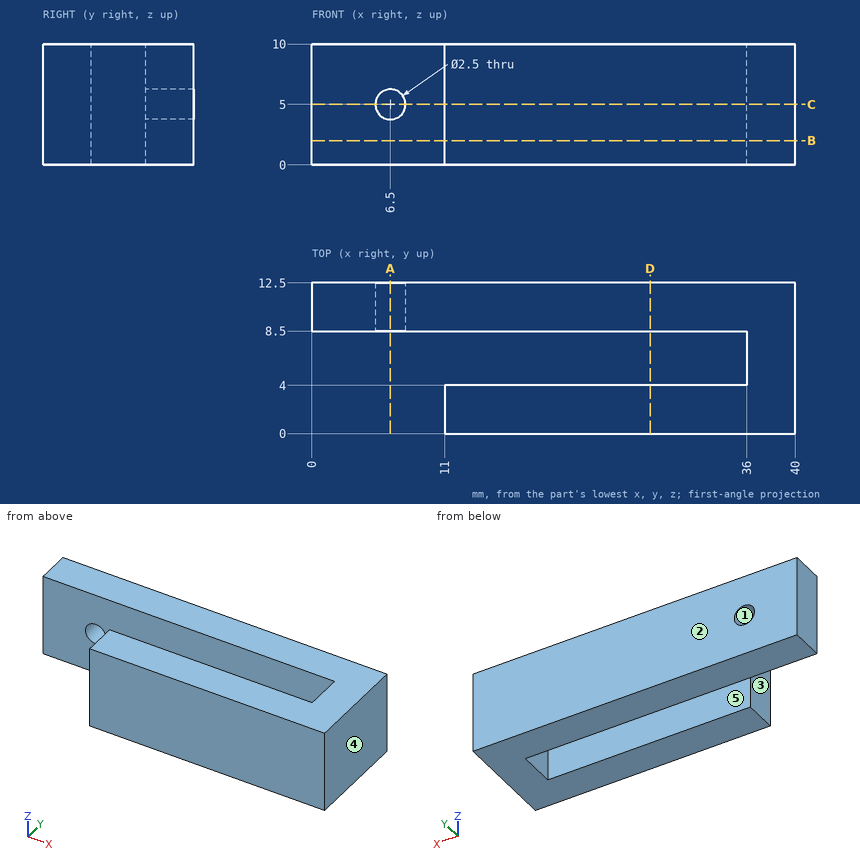
Print and shaded views of the part. All mm, measured from the part's lowest x, y and z. A direction names the side the tool comes from. Give positions to 0.01 mm unless a question says otherwise; leave off trailing zeros. Loops run counter-clockwise (first coordinate to the right, second up) from the corner with the lowest first, then second, coordinate; pieces in that order, holes last. Notation, with made-up numbers: (85, -39) -> (99, -39) arc R16 ccw to (99, -14) -> close; hole circle Ø11 at (15, 52.25). An arc over 180 degrees is marked (long way). Answer in a Markdown table with one row per item.
Item 1: Slice it at B-B on z = 2. Write the cut outline in (x, y).
Findings below:
| item | result |
|---|---|
| outline | (0, 8.5) -> (36, 8.5) -> (36, 4) -> (11, 4) -> (11, 0) -> (40, 0) -> (40, 12.5) -> (0, 12.5) -> close |
Item 2: Slice it at C-C on z = 5. Write the cut outline in (x, y), plus the area to 3 significant figures.
Findings below:
| item | result |
|---|---|
| outline | (0, 8.5) -> (5.25, 8.5) -> (5.25, 12.5) -> (0, 12.5) -> close; (7.75, 8.5) -> (36, 8.5) -> (36, 4) -> (11, 4) -> (11, 0) -> (40, 0) -> (40, 12.5) -> (7.75, 12.5) -> close |
| area | 284 mm² |
Item 3: Slice it at D-D on x = 28. Write the cut outline in (y, z).
Findings below:
| item | result |
|---|---|
| outline | (0, 0) -> (4, 0) -> (4, 10) -> (0, 10) -> close; (8.5, 0) -> (12.5, 0) -> (12.5, 10) -> (8.5, 10) -> close |
Item 4: Flat gauge pins, fed straight in: P1, Ø1, axis at y = 1.5, z = 1, coming from the -X side; P2, Ø1.5, axis at y = 10, z = 1, coming from the -X side; P3, Ø2, axis at y = 6.5, z = 3.5, coming from the -X side; P4, Ø6, axis at x = 4.5, y = 3.5, coming from the +Z side. Where does each tip first touch, or does it go through?
Findings below:
| item | result |
|---|---|
| P1 | stops at x = 11 |
| P2 | stops at x = 0 |
| P3 | stops at x = 36 |
| P4 | passes through |
Item 5: Tool access for the marked faces 4 and 5: list every direction of +Z, -Z, +X, -X, +Y, -Y with a clear straight run to the whole face (end or side of a thin tool).
Findings below:
| item | result |
|---|---|
| face 4 | +Z, -Z, +X, +Y, -Y |
| face 5 | +Z, -Z, -X |
Item 6: Slice it at A-A on x = 6.5. Write the cut outline in (y, z).
Findings below:
| item | result |
|---|---|
| outline | (8.5, 0) -> (12.5, 0) -> (12.5, 3.75) -> (8.5, 3.75) -> close; (8.5, 6.25) -> (12.5, 6.25) -> (12.5, 10) -> (8.5, 10) -> close |
Item 7: Probe line 1 along Z through (x, y) = (6.5, 11.35); line 2 along Y through (x, z) = (13.5, 9.25); line 3 along X through (y, z) = (1.5, 2.25). List the from-to ranges inside material, lowest first. Write a range as [from, to].
Findings below:
| item | result |
|---|---|
| line 1 | z = [0, 3.75], [6.25, 10] |
| line 2 | y = [0, 4], [8.5, 12.5] |
| line 3 | x = [11, 40] |
Item 8: Mould opens along X. For the marked faces 1, 2 and 3 say: pulls with the +X half, pulls with the -X half, needs draft (parallel to the pull), parting line crosses it, or undercut.
Findings below:
| item | result |
|---|---|
| face 1 | undercut |
| face 2 | needs draft |
| face 3 | pulls with the -X half |
